Autodesk Inventor part; units mm, degrees
ref_plane "Work Plane4" through (0, 0, 7) normal (0, 0, 1) x (1, 0, 0)
ref_plane "YZ Plane" through (0, 0, 0) normal (1, 0, 0) x (0, 1, 0)
ref_plane "XZ Plane" through (0, 0, 0) normal (0, 1, 0) x (-1, 0, 0)
sketch "Sketch1" plane through (0, 0, 0) normal (0, 1, 0) x (-1, 0, 0)
  circle A0 centre (0, 0) radius 7
  dimension "d0" = 14
extrude "Extrusion1" add sketch "Sketch1" along normal blind 24.5
sketch "Sketch2" plane through (0, 24.5, 0) normal (0, 1, 0) x (1, 0, 0)
  circle A0 centre (0, 0) radius 4
  dimension "d3" = 8
extrude "Extrusion2" cut sketch "Sketch2" against normal blind 12.25
sketch "Sketch3" plane through (0, 0, 0) normal (0, -1, 0) x (1, 0, 0)
  circle A0 centre (0, 0) radius 2.5
  dimension "d6" = 5
extrude "Extrusion3" cut sketch "Sketch3" against normal blind 12.25
fillet "Fillet1" radius 0.5 4 edges at (7, 24.5, 0) (7, 0, 0) (-4, 24.5, 0) (-2.5, 0, 0)
ref_plane "Work Plane4" through (0, 0, 7) normal (0, 0, 1) x (1, 0, 0)
sketch "Sketch8" plane through (0, 0, 7) normal (0, 0, 1) x (1, 0, 0)
  line L0 (0, 0) -> (0, 24.5) construction
  circle A0 centre (0, 5) radius 1.5
  circle A1 centre (0, 19.5) radius 1.5
  line L1 (-6.5, 24.5) -> (6.5, 24.5)
  dimension "d33" = 3
  dimension "d34" = 5
  dimension "d38" = 5
hole "Hole3" at (0, 5, 7) at (0, 19.5, 7) direction (0, 0, -1) diameter 3.242 end through all
properties part number "Rigid_Coupler" material "Aluminum 6061"
Source: CAD feature listing. Evaluate the final solid. Frame: model axes, mm. A direction names the side the tool comes from. Give positions to 0.01 mm unless a question says otherwise; leave off trailing zeros. Write each loop counter-clockwise with the first axis right and the second up, starting at its lowest first coordinate (ties: lowest second). Pieces come first, ordered by that corner, then holes.
1. Pull-direction query (Z, two-part tool) for faces 1 (the face through (2.31, 6.29, -0.96)), 2 (the face through (-3.23, 12.09, 6.21)), 3 (the face through (1.54, 24.5, 4.42)); classes: +Z half, -Z half, draft (parallel to the pull), parting line (faces both ways), or undercut.
2. Section query C-C (y = 8). Return the cut outline in (x, z).
3. Section query A-A (z = 0). Return the cut outline in (x, y), then the cut area to 3 significant figures.
4. Section query D-D (x = 0). Count the separate pieces of the cut face and the enclosed holes in it, then the cut area to 3 significant figures.
5. Access query for faces 4 (the face through (2, 12.25, -2)), 5 (the face through (-3, 0, -1)). Directions: +Z, -Z, +X, -X, +Y, -Y. A direction counts if a zero-diameter tool reaches every point of the face in a straight line with its end or side. Return the directions, or none.
6. First-contact query: pin 1 (4 mm diameter, centred on x = 0.5, z = -1, fed in from +Y); pin 2 (8 mm diameter, centred on x = 5, y = 12, fed in from -Z); pin 3 (4 mm diameter, centred on y = 6.5, z = -2.5, fed in from +X). Flat tips, straight axial feed; report the tip coordinate or a pass-through.
7. Material intervals for line 1 along Y through (x, z) = (0, 5.05); line 2 along Y through (x, z) = (-1.25, -6); line 3 along Z through (x, y) = (0.5, 2.75), sorted ascending.
8. Section query B-B (y = 20.5). Return the cut outline in (x, z), then the cut area to 3 significant figures.
Output values:
1. face 1: undercut
1. face 2: parting line
1. face 3: draft
2. outline: circle Ø14 at (0, 0); hole circle Ø5 at (0, 0)
3. outline: (-7, 0.5) arc R0.5 ccw to (-6.5, 0) - (-3, 0) arc R0.5 ccw to (-2.5, 0.5) - (-2.5, 12.25) - (-4, 12.25) - (-4, 24) arc R0.5 ccw to (-4.5, 24.5) - (-6.5, 24.5) arc R0.5 ccw to (-7, 24) - close; (2.5, 0.5) arc R0.5 ccw to (3, 0) - (6.5, 0) arc R0.5 ccw to (7, 0.5) - (7, 24) arc R0.5 ccw to (6.5, 24.5) - (4.5, 24.5) arc R0.5 ccw to (4, 24) - (4, 12.25) - (2.5, 12.25) - close
3. area: 183 mm2
4. separate pieces: 6
4. enclosed holes: 0
4. area: 135 mm2
5. face 4: +Y
5. face 5: +Z, -Z, +X, -X, -Y
6. pin 1: stops at y = 12.25
6. pin 2: stops at z = -6.93
6. pin 3: stops at x = 6.98
7. line 1: y = 0 to 3.38, 6.62 to 17.88, 21.12 to 24.5
7. line 2: y = 0 to 3.97, 6.03 to 18.47, 20.53 to 24.5
7. line 3: z = -6.98 to -2.45, 2.45 to 6.98
8. outline: (-1.28, -6.88) - (-1.28, -3.79) arc R4 cw to (-1.28, 3.79) - (-1.28, 6.88) arc R7 ccw to start; (1.28, -6.88) arc R7 ccw to (1.28, 6.88) - (1.28, 3.79) arc R4 cw to (1.28, -3.79) - close
8. area: 88.2 mm2
